Can you work these out from the model? Positions are in its coordinate system, mm. A direction names the side the tool comes from. Round coordinates to 2 decimals unless told otherwise and drop trailing zeros. Order: outer loops, then holes, each group sorted by start corner. A loop starts at its lowest first (then second) coordinate and runs counter-clockwise, first axis right, second up. Notation, with made-up numbers: (84.5, 72.25) -> (132.5, 72.25) arc R18 cw to (132.5, 103.25) -> close; hole circle Ø10 at (-35.5, 77). An arc over 180 degrees is marked (long way). One line per item, written item: value.
Autodesk Inventor part; units mm, degrees
ref_plane "Work Plane1" through (10, 0, 0) normal (0, 0, 1) x (1, 0, 0)
ref_plane "YZ Plane" through (0, 0, 0) normal (1, 0, 0) x (0, 1, 0)
ref_plane "XZ Plane" through (0, 0, 0) normal (0, 1, 0) x (-1, 0, 0)
sketch "Sketch1" plane through (0, 0, 0) normal (0, 0, 1) x (1, 0, 0)
  line L0 (0, 0) -> (10, 0)
  line L1 (20, 3.4641) -> (20, 6)
  line L2 (20, 6) -> (0, 6)
  line L3 (20, 3.4641) -> (12, 3.4641)
  line L4 (12, 3.4641) -> (10, 0)
  line L5 (0, -1.2) -> (0, 7.2)
  line L6 (0, 6) -> (0, 0)
  dimension "d0" = 8
  dimension "d1" = 60
  dimension "d2" = 12
  dimension "d3" = 6.9282
  dimension "d5" = 20
revolve "Body" add sketch "Sketch1" angle 360 about axis through (0, 0, 0) along (1, 0, 0)
sketch "Sketch2" plane through (20, 0, 0) normal (1, 0, 0) x (0, 1, 0)
  circle A0 centre (0, 0) radius 3.4641
  line L0 (-1.7321, 3) -> (1.7321, 3)
  line L1 (1.7321, 3) -> (3.4641, 0)
  line L2 (3.4641, 0) -> (1.7321, -3)
  line L3 (1.7321, -3) -> (-1.7321, -3)
  line L4 (-1.7321, -3) -> (-3.4641, 0)
  line L5 (-3.4641, 0) -> (-1.7321, 3)
  point P0 (0, 0)
  point P1 (0, 0)
extrude "Slot" add sketch "Sketch2" against normal up to next contours L1 A0 | A0 L2 | L0 A0 | A0 L3 | L5 A0 | A0 L4
thread "Thread"
chamfer "Chamfer1" distance 1.0735 angle 45 1 edges at (20, -6, 0) measured on face at (13.3333, 5.9805, -0.4828)
chamfer "Chamfer2" distance 1.0735 angle 45 1 edges at (0, -6, 0) measured on face at (6.3088, 5.9805, -0.4828)
ref_plane "Work Plane1" through (10, 0, 0) normal (0, 0, 1) x (1, 0, 0)
equation "\"d8\" = NLG"
equation "\"d10\" = -0.5 * GD1 + 0.5 * NND"
equation "\"d11\" = FAWI"
equation "\"d34\" = -0.5 * GD1 + 0.5 * NND"
equation "\"d12\" = -0.5 * GD1 + 0.5 * NND"
equation "\"d13\" = FAWI"
equation "\"d35\" = -0.5 * GD1 + 0.5 * NND"
equation "\"d0\" = INTI"
equation "\"d2\" = NND"
equation "\"d3\" = 1.1547 * SW"
equation "\"d5\" = NLG"
equation "\"NND\" = 12"
equation "\"NLG\" = 20"
equation "\"INTI\" = 8"
equation "\"FAWI\" = 45deg"
equation "\"SW\" = 6"
equation "\"GD1\" = THREADDIA - 1.2269 * PTC"
equation "\"SPD\" = 8.5"
equation "\"GUL\" = 0.61345 * PTC"
equation "\"TOA\" = 30deg"
equation "\"THREADDIA\" = 12"
equation "\"PTC\" = 1.75"
equation "\"FAWI1\" = 45deg"
equation "\"GAL\" = 0.61345 * PTC"
equation "\"E0\" = 1.155 * SW"
properties part number "DIN 913 - M12 x 20" material "Steel, Mild"
Q1. On a 3-axis mill with a long thin cutter (end or side, diameter ignored), from which of +Z, -Z, +X, -X, +Y, -Y can I reach the whole of each face in a straight line? I mean faces 1 (the face through (16, 0, 3)), 2 (the face through (0, 0, 0)). Say none if no direction works.
Answers below:
face 1: +X
face 2: +Z, -Z, -X, +Y, -Y
Q2. We'd pull the mould along Z, two halves only. Please class faces 3 (the face through (10, -6, 0)), 4 (the face through (15.9, 2.6, 1.5)), 5 (the face through (20, -0.1, -3.2)), 6 (the face through (15.9, -2.6, -1.5)): released by +Z, released by -Z, zero draft, split by the parting line, or undercut.
Answers below:
face 3: split by the parting line
face 4: undercut
face 5: zero draft
face 6: undercut
Q3. Please list where these lines run through material, in increasing order: line 1 along Z through (x, y) = (8.5, 0.25); line 2 along Y through (x, z) = (17.75, 0.25); line 3 along Y through (x, z) = (8.75, -4.75).
Answers below:
line 1: -5.99 to 5.99
line 2: -5.99 to -3.32, 3.32 to 5.99
line 3: -3.67 to 3.67
Q4. I want a section at B-B on x = 6. List the corners of the cut face in (y, z) for me, plus the area to 3 significant figures.
Answers below:
outline: circle Ø12 at (0, 0)
area: 113 mm^2
Q5. Will this pin go through, and if not, where does the flat tip stop? pin 1 Ø1.5 at (x, y) = (15.5, -2.5) entering from -Z.
Answers below:
pin 1: z = -5.74
Q6. I want a section at A-A on x = 15. List the corners of the cut face in (y, z) for me, plus the area to 3 significant figures.
Answers below:
outline: circle Ø12 at (0, 0); hole (-3.46, 0) -> (-1.73, -3) -> (1.73, -3) -> (3.46, 0) -> (1.73, 3) -> (-1.73, 3) -> close
area: 81.9 mm^2
